Autodesk Inventor part; units mm, degrees
ref_plane "YZ Plane" through (0, 0, 0) normal (1, 0, 0) x (0, 1, 0)
ref_plane "XZ Plane" through (0, 0, 0) normal (0, 1, 0) x (-1, 0, 0)
ref_plane "XY Plane" through (0, 0, 0) normal (0, 0, 1) x (1, 0, 0)
sketch "Sketch8" plane through (0, 0, 0) normal (0, 0, 1) x (1, 0, 0)
  line L0 (26.5434, 0) -> (-0.4566, 0)
  line L1 (-0.4566, 0) -> (-0.4566, 13)
  line L2 (-47.4566, 0) -> (-61.4566, 0)
  line L3 (-61.4566, 3) -> (-48.4566, 3)
  line L4 (-29.793, 16) -> (2.5434, 16)
  line L5 (2.5434, 16) -> (2.5434, 3)
  line L6 (2.5434, 3) -> (26.5434, 3)
  line L7 (-61.4566, 0) -> (-61.4566, 3)
  line L8 (26.5434, 3) -> (26.5434, 0)
  line L9 (-29.4566, 30.4084) -> (-29.4566, -16.4271)
  arc A0 (-29.4566, 13) -> (-30.0706, 12.9895) centre (-29.4566, -5) ccw
  arc A1 (-30.0706, 12.9895) -> (-41.3988, 3.4923) centre (-29.6612, 0.9965) ccw
  arc A2 (-48.4566, 3) -> (-44.0702, 5.6) centre (-48.4566, 8) ccw
  line L10 (-0.4566, 13) -> (-29.4566, 13)
  arc A3 (-47.4566, 0) -> (-41.3988, 3.4923) centre (-47.4566, 7) ccw
  arc A4 (-29.793, 16) -> (-44.0702, 5.6) centre (-29.793, 1) ccw
  point P0 (0, 0)
  point P1 (-36.7292, 11.4654)
  point P2 (-29.4566, -11.7979)
  dimension "d92" = 88
  dimension "d93" = 27
  dimension "d95" = 16
  dimension "d100" = 3
  dimension "d101" = 3
  dimension "d104" = 14
  dimension "d105" = 13
  dimension "d106" = 32
  dimension "d109" = 5
  dimension "d111" = 12
  dimension "d112" = 7
  dimension "d113" = 3
  dimension "d114" = 15
extrude "Extrusion8" add sketch "Sketch8" along normal mid plane 31
sketch "Sketch9" plane through (-29.793, 16, 15.5) normal (0, 1, 0) x (1, 0, 0)
  line L0 (0, 0) -> (0, 31)
  line L1 (32.3364, 0) -> (0, 0)
  line L2 (0, 31) -> (32.3364, 31)
  arc A0 (8.6831, 6.377) -> (8.6831, 24.0275) centre (7.7775, 15.2022) ccw construction
  line L3 (-3, 28) -> (-3, 3)
  line L4 (-3, 28) -> (21.7382, 28)
  line L5 (-3, 3) -> (21.7382, 3)
  arc A1 (25.1271, 4.875) -> (25.1271, 26.125) centre (8.1828, 15.5) ccw
  arc A2 (25.1271, 26.125) -> (21.7382, 28) centre (21.7382, 24) ccw
  arc A3 (21.7382, 3) -> (25.1271, 4.875) centre (21.7382, 7) ccw
  point P0 (29.793, 15.5)
  point P1 (23.7953, 28)
  point P2 (23.7953, 3)
  dimension "d115" = 3
  dimension "d116" = 3
  dimension "d117" = 3
  dimension "d118" = 20
  dimension "d119" = 4
extrude "Extrusion9" cut sketch "Sketch9" against normal blind 4
sketch "Sketch10" plane through (2.5434, 3, 15.5) normal (0, 1, 0) x (1, 0, 0)
  line L0 (24, 0) -> (24, 31)
  line L1 (0, 31) -> (24, 31)
  circle A0 centre (12.8467, 12.1299) radius 2.4585
  circle A1 centre (-59.1533, 12.1299) radius 2.4585
  line L2 (24, 15.5) -> (-63.997, 15.5) construction
  line L3 (12.8467, 12.1299) -> (12.8467, 22.8922)
  line L4 (-59.1533, 12.1299) -> (-59.1533, 22.8922)
  point P0 (-2.5434, 15.5)
  point P1 (-59.1533, 15.5)
  point P2 (12.8467, 15.5)
hole "Hole1" at (-56.6099, 3, 0) at (15.3901, 3, 0) direction (0, -1, 0) diameter 6 depth 5 tip angle 118
sketch "Sketch11" plane through (2.5434, 3, 15.5) normal (0, 1, 0) x (1, 0, 0)
  circle A0 centre (12.8467, 15.5) radius 3
  line L0 (24, 0) -> (0, 0)
  line L1 (12.8467, 15.5) -> (37.9107, 15.5) construction
  line L2 (12.8467, 12.5) -> (37.9107, 12.5)
  line L3 (37.9107, 18.5) -> (12.8467, 18.5)
  arc A1 (12.8467, 18.5) -> (12.8467, 12.5) centre (12.8467, 15.5) ccw
  arc A2 (37.9107, 12.5) -> (37.9107, 18.5) centre (37.9107, 15.5) ccw
  circle A3 centre (-59.1533, 15.5) radius 3
  line L4 (-59.1533, 15.5) -> (-73.4296, 15.5) construction
  line L5 (-59.1533, 12.5) -> (-73.4296, 12.5)
  line L6 (-73.4296, 18.5) -> (-59.1533, 18.5)
  arc A4 (-59.1533, 12.5) -> (-59.1533, 18.5) centre (-59.1533, 15.5) ccw
  arc A5 (-73.4296, 18.5) -> (-73.4296, 12.5) centre (-73.4296, 15.5) ccw
  point P0 (-2.5434, 15.5)
  point P1 (25.3787, 15.5)
  point P2 (-66.2914, 15.5)
extrude "Extrusion10" cut sketch "Sketch11" against normal blind 4 contours A0 L3 A2 L2 | A3 | A3 L5 A5 L6
chamfer "Chamfer1" distance 10 angle 45 4 edges at (26.5434, 1.5, 15.5) (-61.4566, 1.5, 15.5) (-61.4566, 1.5, -15.5) (26.5434, 1.5, -15.5)
equation "\"d2\" = 0.5 * d1"
equation "\"d3\" = 0.5 * d0"
properties part number "SUPPORT PLSTE" material "Stainless Steel, 440C"
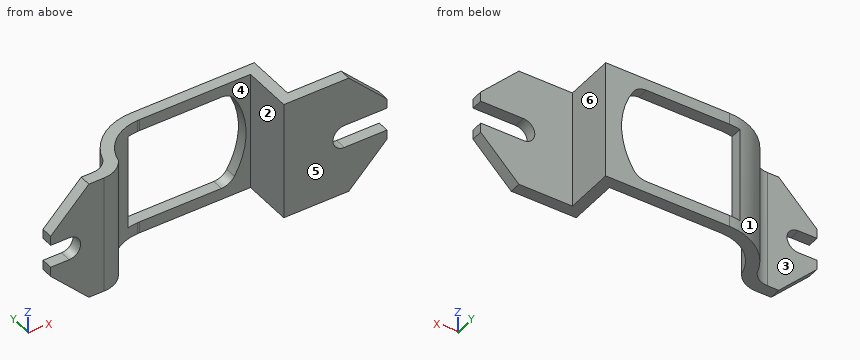
Part model, mm, in its own coordinate system. Face numbers are marked on the shaded views. A direction names the side the tool comes from. Coordinates: 2 decimals unless noted, no trailing zeros. Write each loop counter-clockwise with the first axis right and the second up, starting at its lowest first coordinate (ties: lowest second). Pieces come first, ordered by that corner, then holes. Notation, with made-up numbers: M -4.75,-19 L 11.25,-19 A18 cw 11.25,-10 Z; hole C 65.25,81 d7. An arc over 180 degrees is marked long. Return JSON: item names as keys, results as strings.
1. Saw through at A-A, the plane x = -17.5. Write the cut outline in (y, z), then the cut area to 3 significant figures.
Determined:
{"outline": "M 13,-15.5 L 16,-15.5 L 16,-12.5 L 13,-12.5 Z; M 13,12.5 L 16,12.5 L 16,15.5 L 13,15.5 Z", "area": "18.0 mm²"}
2. Flat gauge pins, fed straight in: pin 1 Ø8 at (x, y) = (-16, 8) entering from +Z; pin 2 Ø3.5 at (x, y) = (-59.5, 1.5) entering from -Z; pin 3 Ø0.9 at (x, y) = (-58.5, 2) entering from +Z; pin 4 Ø1.5 at (x, y) = (18.5, 1.5) entering from -Z. Where does each tip first touch, or does it go through?
Determined:
{"pin 1": "through", "pin 2": "z = -9.21", "pin 3": "z = 8.91", "pin 4": "z = -14.29"}
3. Probe L1, parallel to X at y = 2, z = 4; L2, parallel to X at y = 2.75, z = -5; L3, parallel to Y at x = -14.5, z = 14. List the from-to ranges inside material, lowest first.
Determined:
{"L1": "-61.46 to -42.56, -0.46 to 26.54", "L2": "-61.46 to -41.89, -0.46 to 26.54", "L3": "13 to 16"}
4. 3-axis set-ups, long thin cutter, end or side, ignore diameter. For the marked faces 4, 5 and 6: which of +Z, -Z, +X, -X, +Y, -Y reach the whole face in a straight line?
Determined:
{"face 4": "+Z, -Z, -Y", "face 5": "+Z, -Z, +X, -X, -Y", "face 6": "+Z, -Z, +X, +Y"}
5. Saw through at D-D, the plane y = 14.75. Write the cut outline in (x, z) (3 decimals), then the cut area to 3 significant figures.
Determined:
{"outline": "M -35.788,-15.5 L 2.543,-15.5 L 2.543,15.5 L -35.788,15.5 Z; hole M -32.793,-12.5 L -8.055,-12.5 A4 ccw -4.666,-10.625 A20 ccw -4.666,10.625 A4 ccw -8.055,12.5 L -32.793,12.5 Z", "area": "445 mm²"}
6. Pull direction X, two halves, no side cores. Call the marked faces 1, 2 and 3: pulls with the +X half, pulls with the -X half, needs draft (parallel to the pull), parting line crosses it, or undercut.
Determined:
{"face 1": "pulls with the -X half", "face 2": "undercut", "face 3": "needs draft"}
7. Saw through at B-B, the plane z = 0. Write the cut outline in (x, y), then the cut area to 3 significant figures.
Determined:
{"outline": "M -53.61,0 L -47.46,0 A7 ccw -41.4,3.49 A12 cw -32.79,12.58 L -32.79,15.7 A15 ccw -44.07,5.6 A5 cw -48.46,3 L -53.61,3 Z; M -1.61,13 L -0.46,13 L -0.46,0 L 12.39,0 L 12.39,3 L 2.54,3 L 2.54,16 L -1.61,16 Z", "area": "164 mm²"}
8. Saw through at C-C, the plane y = 10. Write the cut outline in (x, z), then the cut area to 3 significant figures.
Determined:
{"outline": "M -41.79,-15.5 L -37.59,-15.5 L -37.59,15.5 L -41.79,15.5 Z; M -0.46,-15.5 L 2.54,-15.5 L 2.54,15.5 L -0.46,15.5 Z", "area": "223 mm²"}
